Verification items for the finished model (mm, model axes). Face numbers are marked on the shaded views. Coordinates: 2 decimals unless noted, no trailing zeros. Order: outer loops, then holes, each group sorted by start corner. A loop starts at its lowest first (then second) coordinate and runs counter-clockwise, first axis right, second up. Notation, with made-up numbers: (20.25, -19.75) -> (46.25, -19.75) arc R15 cw to (46.25, 9.25) -> close; hole circle Ø3 at (15, 44). An arc over 180 degrees is marked (long way). Use CSV: the item, a comma, the result in double quotes. Start each with the question number.
1) Sectioned sample at C-C on z = 165.5. Record the boundary of the cut face in (x, y).
2) Sectioned sample at B-B on x = -785. Record the boundary of the cut face in (y, z) (3 decimals).
3) Scan lines: line 1 along X through (y, z) = (-4, 95); line 2 along Z through (x, y) = (-330, -15.5) (3 decimals); line 3 along Y through (x, z) = (-624, 78). Record each from-to range of solid material in increasing order.
4) Sectioned sample at A-A on y = -25.5. Record the boundary of the cut face in (x, z) (3 decimals).
5) Release check for a two-part mould opening along Z. For the marked faces 1 and 2 record: released by +Z, released by -Z, zero draft, split by the parting line, or undercut.
6) Go/stop test with a flat-tipped pin: pin 1 (10 mm diameter, centred on x = -737, z = -153, fed in from +Y). Record where the tip stops, or that it passes through.
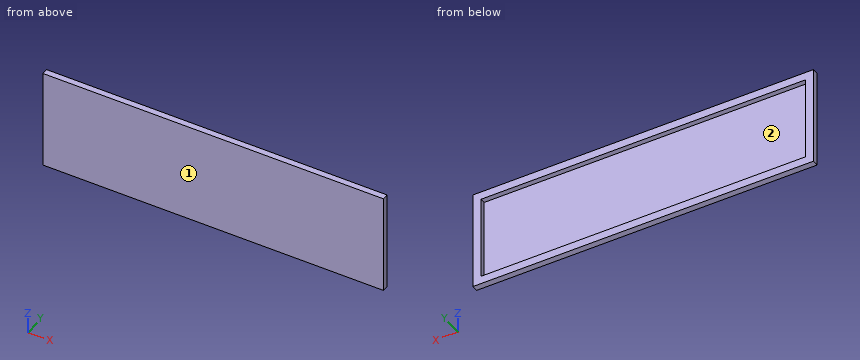
from build123d import *

# Parameters (mm, degrees)
F0_W     = 2118.36
F0_H     = 638.81
F1_DEPTH = 38.1
F2_W     = 2016.76
F2_H     = 537.21
F3_DEPTH = 31.75


with BuildPart() as f1:
    # F0 (on Front) → F1 (new body)
    with BuildSketch(Plane.XZ):
        Rectangle(F0_W, F0_H)
    extrude(amount=F1_DEPTH)

    # F2 (on face) → F3 (cut)
    with BuildSketch(Plane(origin=(0, 0, 0), x_dir=(-1, 0, 0), z_dir=(0, 1, 0))):
        Rectangle(F2_W, F2_H)
    extrude(amount=-F3_DEPTH, mode=Mode.SUBTRACT)


solid = f1.part
Answers follow:
1,outline,"(-1059.18, -38.1) -> (1059.18, -38.1) -> (1059.18, 0) -> (1008.38, 0) -> (1008.38, -31.75) -> (-1008.38, -31.75) -> (-1008.38, 0) -> (-1059.18, 0) -> close"
2,outline,"(-38.1, -319.405) -> (0, -319.405) -> (0, -268.605) -> (-31.75, -268.605) -> (-31.75, 268.605) -> (0, 268.605) -> (0, 319.405) -> (-38.1, 319.405) -> close"
3,line 1,"x = -1059.18 to -1008.38, 1008.38 to 1059.18"
3,line 2,"z = -319.405 to -268.605, 268.605 to 319.405"
3,line 3,"y = -38.1 to -31.75"
4,outline,"(-1059.18, -319.405) -> (1059.18, -319.405) -> (1059.18, 319.405) -> (-1059.18, 319.405) -> close; hole (-1008.38, -268.605) -> (1008.38, -268.605) -> (1008.38, 268.605) -> (-1008.38, 268.605) -> close"
5,face 1,"zero draft"
5,face 2,"undercut"
6,pin 1,"stops at y = -31.75"
